```python
from build123d import *

# Parameters (mm, degrees)
SKETCH_W        = 85
SKETCH_H        = 120
PAD_DEPTH       = 10
SKETCH001_R     = 2.6
POCKET_DEPTH    = 10
SKETCH002_W     = 85
SKETCH002_H     = 28
POCKET001_DEPTH = 5
SKETCH003_W     = 10
SKETCH003_H     = 20
PAD001_DEPTH    = 12
SKETCH004_R     = 1.7
SKETCH004_W     = 6
SKETCH004_H     = 2
POCKET002_DEPTH = 10
SKETCH005_R     = 1.7
SKETCH005_W     = 6
SKETCH005_H     = 2
POCKET003_DEPTH = 10


with BuildPart() as part:
    # Sketch → Pad (new body)
    with BuildSketch(Plane.YZ):
        with Locations((42.5, 60)):
            Rectangle(SKETCH_W, SKETCH_H)
    extrude(amount=PAD_DEPTH)

    # Sketch001 (on Face6 of Pad) → Pocket (cut)
    with BuildSketch(Plane.YZ.offset(10)):
        with Locations((12.496559, 7)):
            Circle(SKETCH001_R)
        with Locations((72.499756, 7)):
            Circle(SKETCH001_R)
        with Locations((12.498186, 43)):
            Circle(SKETCH001_R)
        with Locations((72.504387, 43)):
            Circle(SKETCH001_R)
        with Locations((12.483372, 113)):
            Circle(SKETCH001_R)
        with Locations((72.5, 113)):
            Circle(SKETCH001_R)
        with Locations((72.5, 77)):
            Circle(SKETCH001_R)
        with Locations((12.510227, 77)):
            Circle(SKETCH001_R)
    extrude(amount=-POCKET_DEPTH, mode=Mode.SUBTRACT)

    # Sketch002 (on Face5 of Pocket) → Pocket001 (cut)
    with BuildSketch(Plane.YZ.offset(10)):
        with Locations((42.5, 25)):
            Rectangle(SKETCH002_W, SKETCH002_H)
        with Locations((42.5, 95)):
            Rectangle(SKETCH002_W, SKETCH002_H)
    extrude(amount=-POCKET001_DEPTH, mode=Mode.SUBTRACT)

    # Sketch003 (on Face4 of Pocket001) → Pad001 (join)
    with BuildSketch(Plane(origin=(0, 0, 0), x_dir=(0, 1, 0), z_dir=(-1, 0, 0))):
        with Locations((20, -60)):
            Rectangle(SKETCH003_W, SKETCH003_H)
        with Locations((65, -60)):
            Rectangle(SKETCH003_W, SKETCH003_H)
    extrude(amount=PAD001_DEPTH)

    # Sketch004 (on Face28 of Pad001) → Pocket002 (cut)
    with BuildSketch(Plane(origin=(0, 15, 0), x_dir=(0, 0, -1), z_dir=(0, -1, 0))):
        with Locations((-67, -5)):
            Circle(SKETCH004_R)
        with Locations((-53, -5)):
            Circle(SKETCH004_R)
        with Locations((-60.033646, -1)):
            Rectangle(SKETCH004_W, SKETCH004_H)
        with Locations((-60, -6.999858)):
            Rectangle(SKETCH004_W, SKETCH004_H)
    extrude(amount=-POCKET002_DEPTH, mode=Mode.SUBTRACT)

    # Sketch005 (on Face19 of Pocket002) → Pocket003 (cut)
    with BuildSketch(Plane.ZX.offset(70)):
        with Locations((53, -5)):
            Circle(SKETCH005_R)
        with Locations((67, -5)):
            Circle(SKETCH005_R)
        with Locations((60, -1)):
            Rectangle(SKETCH005_W, SKETCH005_H)
        with Locations((60, -7)):
            Rectangle(SKETCH005_W, SKETCH005_H)
    extrude(amount=-POCKET003_DEPTH, mode=Mode.SUBTRACT)


solid = part.part
```
Could you check a few things on this model? Use its own coordinates, in mm. A direction names the side the tool comes from. Round coordinates to 2 decimals unless told otherwise and drop trailing zeros. Loops run counter-clockwise (first coordinate to the right, second up) from the corner with the lowest first, then second, coordinate; pieces in that order, holes last.
Q1. I want a section at C-C (y = 72.5). Write out the boundary of the cut face in (x, z), and give its area (3 significant figures).
Q2. Please list where these lines run through material, in increasing order: L1, parallel to Z at x = 4.25, y = 72.5; L2, parallel to Y at x = 5, z = 42; L3, parallel to X at y = 76.5, z = 103.5.
Q3. I want a section at A-A (x = 8). Give the number of separate pieces and of enclosed holes in the cut face, and give its area (3 significant figures).
Q4. On a 3-axis mill with a long thin cutter (end or side, diameter ignored), from which of +Z, -Z, +X, -X, +Y, -Y can I reach the whole of each face in a straight line? I mean faces 4 (the flat face through (-2, 20, 60)), 5 (the flat face through (8, 42, 39)), 6 (the flat face through (-12, 65, 60)). Say none if no direction works.
Q5. I want a section at B-B (z = 61.5). Write out the boundary of the cut face in (x, y).
Q6. I want a section at D-D (z = 43). Write out the boundary of the cut face in (x, y).
Q7. For P1, Ø0.6, axis at x = -1, y = 18, coming from the +Z side; P2, Ø8.5, axis at y = 72.5, z = 77, coming from the +X side; P3, Ø10, axis at y = 12, z = 13, coming from the -X side; P4, Ø4, axis at y = 12.51, z = 77, coming from the +X side, each with a flat end and sliding along its axis, tell me the tip position at first contact or that it passes through.
Q8. Thinking about a two-plate mould opening in Z: for faces 1 (the flat face through (-6, 65, 50)), 2 (the flat face through (-6, 20, 60)), 3 (the flat face through (-6, 20, 70)), which applies, pulls with the +Z half, pulls with the -Z half, needs draft (parallel to the pull), parting line crosses it, or undercut?
Answer below:
1. outline: (0, 0) - (10, 0) - (10, 4.4) - (0, 4.4) - close; (0, 9.6) - (10, 9.6) - (10, 11) - (5, 11) - (5, 39) - (10, 39) - (10, 40.4) - (0, 40.4) - close; (0, 45.6) - (10, 45.6) - (10, 74.4) - (0, 74.4) - close; (0, 79.6) - (10, 79.6) - (10, 81) - (5, 81) - (5, 109) - (10, 109) - (10, 110.4) - (0, 110.4) - close; (0, 115.6) - (10, 115.6) - (10, 120) - (0, 120) - close
1. area: 712 mm2
2. L1: z = 0 to 4.4, 9.6 to 40.4, 45.6 to 74.4, 79.6 to 110.4, 115.6 to 120
2. L2: y = 0 to 10.1, 14.9 to 70.1, 74.9 to 85
2. L3: x = 0 to 5
3. separate pieces: 3
3. enclosed holes: 8
3. area: 5,270 mm2
4. face 4: +Y, -Y
4. face 5: +X, +Y, -Y
4. face 6: +Z, -Z, -X, +Y, -Y
5. outline: (-12, 15) - (-8, 15) - (-8, 25) - (-12, 25) - close; (-12, 60) - (-8, 60) - (-8, 70) - (-12, 70) - close; (-6, 15) - (-2, 15) - (-2, 25) - (-6, 25) - close; (-6, 60) - (-2, 60) - (-2, 70) - (-6, 70) - close; (0, 0) - (10, 0) - (10, 85) - (0, 85) - close
6. outline: (0, 0) - (10, 0) - (10, 9.9) - (0, 9.9) - close; (0, 15.1) - (10, 15.1) - (10, 69.9) - (0, 69.9) - close; (0, 75.1) - (10, 75.1) - (10, 85) - (0, 85) - close
7. P1: stops at z = 70
7. P2: stops at x = 10
7. P3: stops at x = 0
7. P4: passes through
8. face 1: pulls with the -Z half
8. face 2: undercut
8. face 3: pulls with the +Z half
